Drawing for the job (mm, zero at the part's lowest x, y, z). Coordinates: 2 decimals unless noted, no trailing zeros. Write each loop counter-clockwise with the first axis right and the second up, starting at its lowest first coordinate (ties: lowest second). Pieces come first, ordered by that corner, then holes. Notation, with made-up numbers: M 7,49 L 59,49 A4 ccw 59,56 Z; hole C 89,22 d6. An arc over 180 degrees is marked long. Use a Markdown table: item, result. Add a question column.
Q1. Slice it at C-C on x = 48. Write the cut outline in (y, z).
Q2. Wall check: L1, parallel to X at y = 50, z = 2.25; L2, parallel to Y at x = 47.5, z = 1.3 (1 decimal); L3, parallel to Y at x = 35.5, z = 1.55. Give the ranges that are in metal, low to high. Write a range as from..to.
Q3. Pin check, flat tip, straight feed: pin 1 Ø0.9 at (x, z) = (6.5, 1.5) entering from +Y. Stop position of the tip, or through.
Q4. Slice it at B-B on y = 3. Write the cut outline in (x, z) (1 decimal), then the cut area to 3 significant figures.
Q5. Mould opens along X. For the marked faces 1, 2 and 3 say: released by +X, released by -X, zero draft, split by the parting line, or undercut.
Q6. Slice it at D-D on y = 44. Write the cut outline in (x, z).
Q7. Slice it at A-A on z = 0.6. Write the cut outline in (x, y) (1 decimal), then the cut area to 3 significant figures.
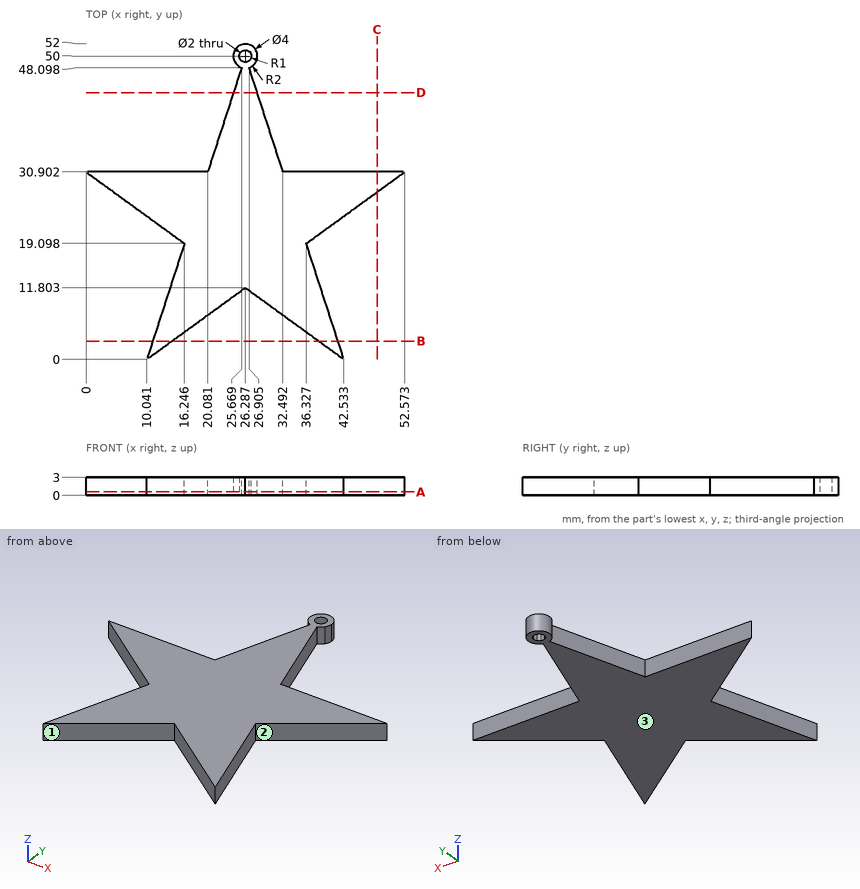
Recorded:
| question | item | result |
|---|---|---|
| 1 | outline | M 27.58,0 L 30.9,0 L 30.9,3 L 27.58,3 Z |
| 2 | L1 | 24.29..25.29, 27.29..28.29 |
| 2 | L2 | 27.2..30.9 |
| 2 | L3 | 5.11..30.9 |
| 3 | pin 1 | y = 30.9 |
| 4 | outline | M 11,0 L 14.2,0 L 14.2,3 L 11,3 Z; M 38.4,0 L 41.6,0 L 41.6,3 L 38.4,3 Z |
| 4 | area | 18.9 mm² |
| 5 | face 1 | undercut |
| 5 | face 2 | released by +X |
| 5 | face 3 | zero draft |
| 6 | outline | M 24.34,0 L 28.24,0 L 28.24,3 L 24.34,3 Z |
| 7 | outline | M 0,30.9 L 16.2,19.1 L 10,0 L 26.3,11.8 L 42.5,0 L 36.3,19.1 L 52.6,30.9 L 32.5,30.9 L 26.9,48.1 A2 ccw long 25.7,48.1 L 20.1,30.9 Z; hole C 26.3,50 d2 |
| 7 | area | 866 mm² |
